Answer from the drawing. Dimensions are ordinates in mm from the lowest x, y and z of the part. A direction names the side the tool comes from. Give positions to 0.01 mm unless a question says otherwise; leave off trailing zeros. Order: outer loops, then holes, each group sorted by start corner. A loop starts at its lowest first (then second) coordinate and runs counter-clockwise, first axis right, second up. Notation, with made-up numbers: (84.5, 76.25) - (114.5, 76.25) arc R22 ccw to (114.5, 100.25) - close; hole circle Ø8 at (79, -24). An arc over 180 degrees is marked (long way). Answer in a Markdown table with one row per item. Add a question column.
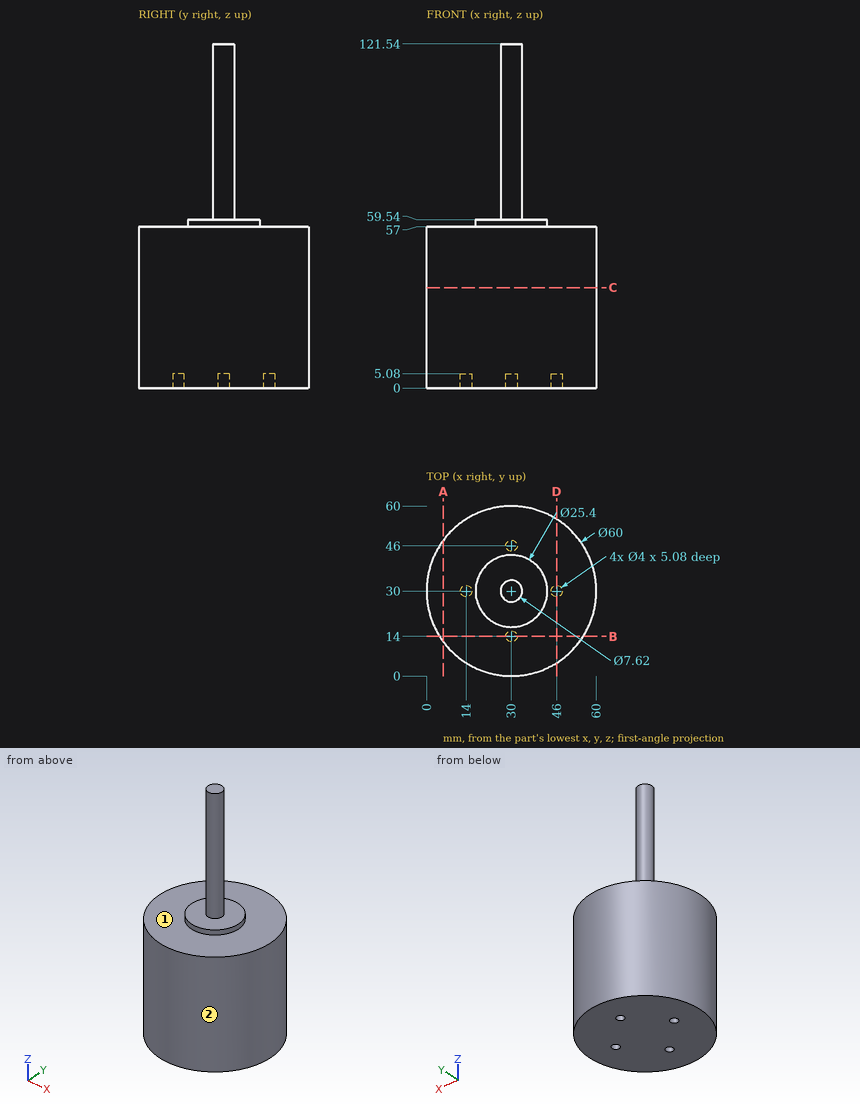
(1) Find section B-B, the plane y = 14. Write down the section's boundary in (x, z), plus the area to 3 significant figures.
(2) For the marked faces 1 and 2, determine the directions among +Z, -Z, +X, -X, +Y, -Y from which every point of the face is accessible in a straight line to the end or side of a thin tool.
(3) Each of these flat-tipped pins is pushed along its axis until it touches: P1, Ø1.5, axis at y = 40.5, z = 28, coming from the +X side; P2, Ø1.5, axis at x = 51.5, y = 27.5, coming from the +Z side; P3, Ø10, axis at x = 52.5, z = 34.5, coming from the -Y side. Where does it stop, or does it pass through?
(4) Find section C-C, the plane z = 35.5. Write down the section's boundary in (x, y), plus the area to 3 significant figures.
(5) Find section A-A, the plane x = 6. Write down the section's boundary in (y, z), plus the area to 3 significant figures.
(6) Straight lines are drawn through the part: line 1 (Z direction, x = 13, y = 22.5); line 2 (Y direction, x = 46, z = 3.45); line 3 (Y direction, x = 50.5, z = 25.5). For each, find the intervals that lie inside material, in ascending order.
Answer key:
| question | item | result |
|---|---|---|
| 1 | outline | (4.62, 0) - (28, 0) - (28, 5.08) - (32, 5.08) - (32, 0) - (55.38, 0) - (55.38, 57) - (4.62, 57) - close |
| 1 | area | 2,870 mm² |
| 2 | face 1 | +Z |
| 2 | face 2 | +Z, -Z |
| 3 | P1 | x = 58.37 |
| 3 | P2 | z = 57 |
| 3 | P3 | y = 5.63 |
| 4 | outline | circle Ø60 at (30, 30) |
| 4 | area | 2,830 mm² |
| 5 | outline | (12, 0) - (48, 0) - (48, 57) - (12, 57) - close |
| 5 | area | 2,050 mm² |
| 6 | line 1 | 0 to 57 |
| 6 | line 2 | 4.62 to 28, 32 to 55.38 |
| 6 | line 3 | 8.1 to 51.9 |
